The listing builds one solid part. Answer for the finished solid, in the listing's coordinates (mm). Coordinates: 2 decimals unless noted, no trailing zeros. Loops run counter-clockwise (first coordinate to the right, second up) from the corner with the lowest first, then second, coordinate; pieces in that order, holes last. Notation, with made-up numbers: (81.25, -15.75) - (133.25, -15.75) arc R29 ccw to (133.25, 23.25) - close; hole circle Ø6 at (87, -30). An arc over 180 degrees is marked (long way). Put each result on its own line as item: value.
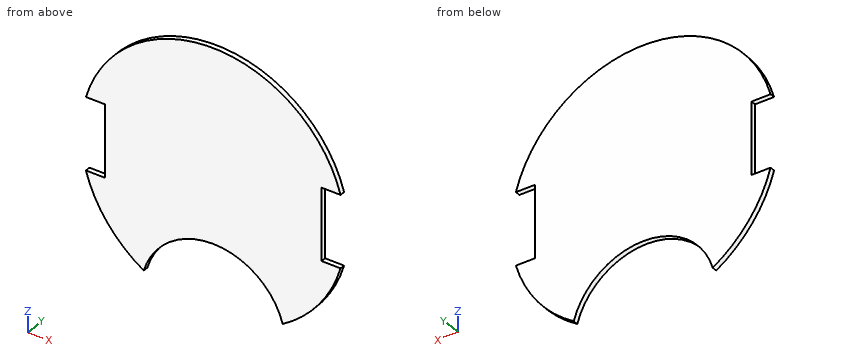
```python
from build123d import *

# Parameters (mm, degrees)
SKETCH2_W           = 279.4
SKETCH2_H           = 279.4
BOSS_EXTRUDE1_DEPTH = 5.334
SKETCH3_OUTSIDE_W   = 360.434
SKETCH3_OUTSIDE_H   = 360.434
CUT_EXTRUDE1_DEPTH  = 198.637626873
SKETCH4_W           = 50.8
SKETCH4_H           = 76.2
CUT_EXTRUDE2_DEPTH  = 198.637626873


with BuildPart() as part:
    # Sketch2 → Boss-Extrude1 (new body)
    with BuildSketch(Plane(origin=(0, 0, 0), x_dir=(1, 0, 0), z_dir=(0, 1, 0))):
        Rectangle(SKETCH2_W, SKETCH2_H)
    extrude(amount=BOSS_EXTRUDE1_DEPTH)

    # Sketch3 outside → Cut-Extrude1 (cut, through all)
    with BuildSketch(Plane(origin=(0, 5.334, 0), x_dir=(1, 0, 0), z_dir=(0, 1, 0))):
        Rectangle(SKETCH3_OUTSIDE_W, SKETCH3_OUTSIDE_H)
        with BuildLine():
            ThreePointArc((-73.311363601, 118.918181818), (0, -139.7), (73.311363601, 118.918181818))
            ThreePointArc((73.311363601, 118.918181818), (0, 63.5), (-73.311363601, 118.918181818))
        make_face(mode=Mode.SUBTRACT)
    extrude(amount=-CUT_EXTRUDE1_DEPTH, mode=Mode.SUBTRACT)

    # Sketch4 → Cut-Extrude2 (cut, through all)
    with BuildSketch(Plane(origin=(0, 5.334, 0), x_dir=(1, 0, 0), z_dir=(0, 1, 0))):
        with Locations((-139.7, 0)):
            Rectangle(SKETCH4_W, SKETCH4_H)
        with Locations((139.7, 0)):
            Rectangle(SKETCH4_W, SKETCH4_H)
    extrude(amount=-CUT_EXTRUDE2_DEPTH, mode=Mode.SUBTRACT)


solid = part.part
```
1) The part is cut by section D-D (x = -85). Give the vertices of the cut face in (y, z), and give its area (3 significant figures).
Found:
outline: (0, -110.87) - (5.33, -110.87) - (5.33, 110.87) - (0, 110.87) - close
area: 1,180 mm^2
2) The part is cut by section C-C (z = -31). Give the vertices of the cut face in (x, y), and give its area (3 significant figures).
Found:
outline: (-114.3, 0) - (114.3, 0) - (114.3, 5.33) - (-114.3, 5.33) - close
area: 1,220 mm^2
3) The part is cut by section A-A (y = 4.3). Give the vertices of the cut face in (x, z), and give its area (3 significant figures).
Found:
outline: (-134.4, -38.1) arc R139.7 ccw to (-73.31, -118.92) arc R76.2 cw to (73.31, -118.92) arc R139.7 ccw to (134.4, -38.1) - (114.3, -38.1) - (114.3, 38.1) - (134.4, 38.1) arc R139.7 ccw to (-134.4, 38.1) - (-114.3, 38.1) - (-114.3, -38.1) - close
area: 49,700 mm^2
4) The part is cut by section B-B (z = -81.5). Give the vertices of the cut face in (x, y).
Found:
outline: (-113.46, 0) - (-49.19, 0) - (-49.19, 5.33) - (-113.46, 5.33) - close; (49.19, 0) - (113.46, 0) - (113.46, 5.33) - (49.19, 5.33) - close
5) Straight lines are drawn through the part: L1, parallel to X at y = 1.9, z = 15.5; L2, parallel to Z at x = 118, y = 2.5; L3, parallel to Z at x = 115, y = 2.8. For each, find the intervals that lie inside material, in ascending order. Write a range as [from, to].
Found:
L1: x = [-114.3, 114.3]
L2: z = [-74.78, -38.1], [38.1, 74.78]
L3: z = [-79.32, -38.1], [38.1, 79.32]
6) Each of these flat-tipped pins is pushed along its axis until it touches: pin 1 (2.5 mm diameter, centred on y = 3, z = -12.5, fed in from -X); pin 2 (2.5 mm diameter, centred on y = 2, z = -14, fed in from +X); pin 3 (3 mm diameter, centred on x = -61.5, y = 3, fed in from -Z). Where does it stop, or does it pass through?
Found:
pin 1: stops at x = -114.3
pin 2: stops at x = 114.3
pin 3: stops at z = -96.83
